For this review, take the finished solid that the model builds, in its own axes (mm). A direction names the side the tool comes from. Give positions to 0.01 mm unless a question says otherwise; leave off trailing zeros. Loops run counter-clockwise (first coordinate to the right, second up) from the corner with the lowest first, then second, coordinate; pieces in that order, holes last. Notation, with made-up numbers: M -17.75,32 L 17.25,32 A25 cw 17.25,71 Z; hole C -10.5,46 d6. An arc over 180 degrees is marked long. Use CSV: the item, a comma, the result in double quotes. Start each with the question number.
1. Take a section at A-A, the plane x = 0. Write out the cut boundary in (y, z).
2. Take a section at D-D, the plane x = -6. Write out the cut boundary in (y, z).
3. The part is to be moulded in two halves that separate along X. For faces 1 (the face through (0, -3, 1.168)), 2 (the face through (0, -1.5, -0.356)), 3 (the face through (-8.25, -2.24, 0.58)), 4 (the face through (-0.032, -3.403, -1.114)), say which applies: pulls with the +X half, pulls with the -X half, needs draft (parallel to the pull), parting line crosses it, or undercut.
4. To check wall thickness, follow line 1 (Z direction, x = -10.5, y = -1.5); line 2 (Y direction, x = 7, z = 0.8); line 3 (X direction, y = 0.5, z = 0.95). State the ranges of each line that lie inside material, in increasing order. Write a range as [from, to].
5. Take a section at C-C, the plane x = 12.5. Write out the cut boundary in (y, z).
6. Take a section at B-B, the plane y = 0. State how many separate pieces and enclosed holes the cut face has, and give its area (3 significant figures).
7. Insertion check: P1, Ø1.6, axis at x = 8, y = 0, coming from the -Z side; P2, Ø1, axis at y = 1.5, z = 0.5, coming from the +X side; P3, Ø4, axis at x = 0, y = 0, coming from the -Z side. Each pin has a flat end and moves straight along its axis. Give the tip position at first contact, or say it passes through.
8. Tool access review of faces 5 (the face through (-0.567, -2.554, 0.542)), 6 (the face through (1.676, 1.536, -1.321)), 7 (the face through (-3.403, 0.043, -1.114)): name each direction out of +Z, -Z, +X, -X, +Y, -Y from which nothing blocks a thin tool from reaching the whole face with its end or side.
Autodesk Inventor part; units mm, degrees
ref_plane "YZ Plane" through (0, 0, 0) normal (1, 0, 0) x (0, 1, 0)
ref_plane "XZ Plane" through (0, 0, 0) normal (0, 1, 0) x (-1, 0, 0)
ref_plane "XY Plane" through (0, 0, 0) normal (0, 0, 1) x (1, 0, 0)
sketch "Sketch1" plane through (0, 0, 0) normal (0, 0, 1) x (1, 0, 0)
  circle A0 centre (0, 0) radius 3.4036
  circle A1 centre (-14.4145, 0) radius 1.8161
  circle A2 centre (14.4145, 0) radius 1.8161
  line L0 (0, 0) -> (0, 12.9246) construction
  line L1 (-14.5375, 1.8119) -> (-2.1305, 2.6543)
  line L2 (2.1305, 2.6543) -> (14.5375, 1.8119)
  line L3 (14.5375, -1.8119) -> (2.1305, -2.6543)
  line L4 (-2.1305, -2.6543) -> (-14.5375, -1.8119)
  dimension "d0" = 6.8072
  dimension "d1" = 3.6322
  dimension "d2" = 32.4612
  dimension "d3" = 5.3086
extrude "Extrusion1" add sketch "Sketch1" along normal blind 1.1684
sketch "Sketch2" plane through (0, 0, 0) normal (0, 0, -1) x (-1, 0, 0)
  arc A0 (14.5375, -1.8119) -> (14.5375, 1.8119) centre (14.4145, 0) ccw
  line L0 (2.1305, 2.6543) -> (14.5375, 1.8119)
  arc A1 (2.1305, 2.6543) -> (-2.1305, 2.6543) centre (0, 0) ccw
  line L1 (-14.5375, 1.8119) -> (-2.1305, 2.6543)
  arc A2 (-14.5375, 1.8119) -> (-14.5375, -1.8119) centre (-14.4145, 0) ccw
  line L2 (-2.1305, -2.6543) -> (-14.5375, -1.8119)
  arc A3 (-2.1305, -2.6543) -> (2.1305, -2.6543) centre (0, 0) ccw
  line L3 (14.5375, -1.8119) -> (2.1305, -2.6543)
  circle A4 centre (0, 0) radius 3.4036
extrude "Extrusion2" add sketch "Sketch2" along normal blind 2.2606 contours A3 A4 A1
sketch "Sketch3" plane through (0, 0, -2.2606) normal (0, 0, -1) x (-1, 0, 0)
  circle A0 centre (0, 0) radius 2.2733
  dimension "d8" = 4.5466
extrude "Extrusion3" cut sketch "Sketch3" against normal blind 1.905
sketch "Sketch4" plane through (0, 0, 1.1684) normal (0, 0, 1) x (1, 0, 0)
  circle A0 centre (0, 0) radius 2.6162
  dimension "d11" = 5.2324
extrude "Extrusion4" cut sketch "Sketch4" against normal blind 1.27
sketch "Sketch5" plane through (0, 0, -0.1016) normal (0, 0, 1) x (1, 0, 0)
  circle A0 centre (0, 0) radius 1.2954
  dimension "d14" = 2.5908
extrude "Extrusion5" cut sketch "Sketch5" against normal blind 1.27
sketch "Sketch6" plane through (0, 0, 1.1684) normal (0, 0, 1) x (1, 0, 0)
  arc A0 (-14.5375, 1.8119) -> (-14.5375, -1.8119) centre (-14.4145, 0) ccw
  circle A1 centre (-14.4145, 0) radius 0.3429
  point P0 (0, 0)
  dimension "d17" = 0.6858
extrude "Extrusion6" cut sketch "Sketch6" against normal through all
pattern_linear "Rectangular Pattern1" count 6 spacing 1.905 along (1, 0, 0) of "Extrusion6"
mirror "Mirror1" about plane through (0, 0, 0) normal (1, 0, 0) of "Extrusion6", "Rectangular Pattern1"
properties part number "2 Way MicroServo Attachment"
Result set:
1,outline,"M -3.4,-2.26 L -2.27,-2.26 L -2.27,-0.36 L -1.3,-0.36 L -1.3,-0.1 L -2.62,-0.1 L -2.62,1.17 L -3.4,1.17 Z; M 1.3,-0.36 L 2.27,-0.36 L 2.27,-2.26 L 3.4,-2.26 L 3.4,1.17 L 2.62,1.17 L 2.62,-0.1 L 1.3,-0.1 Z"
2,outline,"M -2.39,0 L 2.39,0 L 2.39,1.17 L -2.39,1.17 Z"
3,face 1,"needs draft"
3,face 2,"undercut"
3,face 3,"pulls with the -X half"
3,face 4,"parting line crosses it"
4,line 1,"[0, 1.17]"
4,line 2,"[-2.32, -0.27], [0.27, 2.32]"
4,line 3,"[-16.16, -2.57], [2.57, 16.16]"
5,outline,"M -1.95,0 L -0.34,0 L -0.34,1.17 L -1.95,1.17 Z; M 0.34,0 L 1.95,0 L 1.95,1.17 L 0.34,1.17 Z"
6,separate pieces,"14"
6,enclosed holes,"0"
6,area,"27.7 mm2"
7,P1,"z = 0"
7,P2,"x = 15.93"
7,P3,"z = -0.36"
8,face 5,"+Z"
8,face 6,"-Z"
8,face 7,"-Z, -X"
